Autodesk Inventor part; units mm, degrees
ref_plane "YZ Plane" through (0, 0, 0) normal (1, 0, 0) x (0, 1, 0)
ref_plane "XZ Plane" through (0, 0, 0) normal (0, 1, 0) x (-1, 0, 0)
ref_plane "XY Plane" through (0, 0, 0) normal (0, 0, 1) x (1, 0, 0)
sketch "Sketch1" plane through (0, 0, 0) normal (0, 0, 1) x (1, 0, 0)
  circle A0 centre (0, 0) radius 28.575
  circle A1 centre (-23.8125, 0) radius 2.5908
  line L0 (7.3323, 0) -> (3.6662, -6.35)
  line L1 (3.6662, -6.35) -> (-3.6662, -6.35)
  line L2 (-3.6662, -6.35) -> (-7.3323, 0)
  line L3 (-7.3323, 0) -> (-3.6662, 6.35)
  line L4 (-3.6662, 6.35) -> (3.6662, 6.35)
  line L5 (3.6662, 6.35) -> (7.3323, 0)
  line L6 (-23.8125, 0) -> (0, 0) construction
  circle A2 centre (-11.9063, 20.6222) radius 2.5908
  circle A3 centre (11.9062, 20.6222) radius 2.5908
  circle A4 centre (23.8125, 0) radius 2.5908
  circle A5 centre (11.9063, -20.6222) radius 2.5908
  circle A6 centre (-11.9062, -20.6222) radius 2.5908
  dimension "d0" = 57.15
  dimension "d1" = 5.1816
  dimension "d2" = 12.7
  dimension "d3" = 23.8125
  dimension "d6" = 360
extrude "Extrusion1" add sketch "Sketch1" along normal blind 4.572
properties part number "Custom Hex Hub" material "Steel"
The model under review builds one solid part; all positions refer to its coordinate system, in mm. A direction names the side the tool comes from. Coordinates: 2 decimals unless noted, no trailing zeros. Write each loop counter-clockwise with the first axis right and the second up, starting at its lowest first coordinate (ties: lowest second). Pieces come first, ordered by that corner, then holes. Notation, with made-up numbers: (42.5, -4.75) - (53.5, -4.75) arc R30 cw to (53.5, 32.25) - close; hole circle Ø9 at (-5.75, 7.5). An arc over 180 degrees is marked (long way). Answer as a JSON object with one key per item and string values. Group by question number.
1. Mouldability with a two-part tool opening along Y and no side actions: class faces 3 (the face through (5.474, 3.219, 2.254)), 4 (the face through (-28.547, -1.256, 2.254)), 5 (the face through (0, 7, 0)) as pulls with the +Y half, pulls with the -Y half, needs draft (parallel to the pull), parting line crosses it, or undercut.
2. Machinability: for faces 1 (the face through (0, 7, 4.572)), 2 (the face through (-5.474, -3.219, 2.254)), which of the approach directions +Z, -Z, +X, -X, +Y, -Y give a long, thin tool a straight path to every point of the face, cutting with its end or side? Answer none if there is none.
3. Add section D-D (x = -17). Give the boundary of the cut face in (y, z), plus the area to 3 significant figures.
4. Clearance check with flat-ended pins moving along their axes: pin 1 Ø2 at (x, z) = (-9, 3.5) entering from -Y; pin 2 Ø6.5 at (x, y) = (-11.91, 20.62) entering from -Z; pin 3 Ø4 at (x, y) = (11.91, 20.62) entering from +Z; pin 4 Ø1 at (x, z) = (9, 3.5) entering from -Y. State where each tip first meets the part, or that it passes through.
5. To check wall thickness, follow probe 1 along Y at (x, z) = (0, 2.05) (3 decimals); probe 2 along Y at (x, z) = (-14, 4.15); probe 3 along Y at (x, z) = (13.5, 2.4). State the ranges of each line that lie inside material, in increasing order.
6. Add section C-C (y = 24.5). Give the boundary of the cut face in (x, z).
7. Add section A-A (x = 0). Give the boundary of the cut face in (y, z) (3 decimals).
8. Add section B-B (z = 2.5). Give the number of separate pieces and of enclosed holes in the cut face, plus the area to 3 significant figures.
Findings:
{
 "1": {"face 3": "undercut", "face 4": "parting line crosses it", "face 5": "needs draft"},
 "2": {"face 1": "+Z, +X, -X, +Y, -Y", "face 2": "+Z, -Z"},
 "3": {"outline": "(-22.97, 0) - (22.97, 0) - (22.97, 4.57) - (-22.97, 4.57) - close", "area": "210 mm²"},
 "4": {"pin 1": "y = -27.43", "pin 2": "z = 0", "pin 3": "through", "pin 4": "y = -27.28"},
 "5": {"probe 1": "-28.575 to -6.35, 6.35 to 28.575", "probe 2": "-24.91 to -22.15, -19.1 to 19.1, 22.15 to 24.91", "probe 3": "-25.18 to -22.66, -18.58 to 18.58, 22.66 to 25.18"},
 "6": {"outline": "(-14.71, 0) - (14.71, 0) - (14.71, 4.57) - (-14.71, 4.57) - close"},
 "7": {"outline": "(-28.575, 0) - (-6.35, 0) - (-6.35, 4.572) - (-28.575, 4.572) - close; (6.35, 0) - (28.575, 0) - (28.575, 4.572) - (6.35, 4.572) - close"},
 "8": {"separate pieces": "1", "enclosed holes": "7", "area": "2,300 mm²"}
}
